Geometry check sheet. Reference: the model listing, model coordinates, mm. A direction names the side the tool comes from. Round coordinates to 2 decimals unless told otherwise and drop trailing zeros. Write each loop counter-clockwise with the first axis right and the second up, starting at its lowest first coordinate (ties: lowest second). Pieces come first, ordered by that corner, then holes. Notation, with made-up numbers: M -6,83 L 45,83 A5 ccw 45,88 Z; hole C 80,50.25 d5. An arc over 180 degrees is marked long. Use a Markdown table: item, result.
Autodesk Inventor part; units mm, degrees
ref_plane "Work Plane1" through (1.525, 0, 0) normal (0, 0, 1) x (1, 0, 0)
ref_plane "YZ Plane" through (0, 0, 0) normal (1, 0, 0) x (0, 1, 0)
ref_plane "XZ Plane" through (0, 0, 0) normal (0, 1, 0) x (-1, 0, 0)
sketch "Sketch1" plane through (0, 0, 0) normal (0, 0, 1) x (1, 0, 0)
  line L0 (0, 7.1374) -> (0, 4.9276)
  line L1 (101.6, 4.7625) -> (127, 4.7625)
  line L2 (127, 4.7625) -> (127, 0)
  line L3 (127, 0) -> (-0.0001, 0)
  line L4 (-25.4001, 0) -> (152.4, 0)
  line L5 (-0.0001, 0) -> (-0.0001, 7.1374)
  line L6 (-0.0001, 7.1374) -> (0, 7.1374)
  line L7 (101.6, 4.7625) -> (97.6311, 4.9276)
  line L8 (97.6311, 4.9276) -> (0, 4.9276)
  line L9 (0, -1.4275) -> (0, 8.5649)
  dimension "d0" = 127
  dimension "d1" = 25.4
  dimension "d2" = 9.525
  dimension "d9" = 0.0001
  dimension "d10" = 14.2748
  dimension "d13" = 3.9689
  dimension "d14" = 9.8552
revolve "Body" add sketch "Sketch1" angle 360 about axis through (127, 0, 0) along (-1, 0, 0)
sketch "Sketch2" plane through (-0.0001, 0, 0) normal (-1, 0, 0) x (0, 0, 1)
  line L0 (0, 8.2416) -> (7.1374, 4.1208)
  line L1 (7.1374, 4.1208) -> (7.1374, -4.1208)
  line L2 (7.1374, -4.1208) -> (0, -8.2416)
  line L3 (0, -8.2416) -> (-7.1374, -4.1208)
  line L4 (-7.1374, -4.1208) -> (-7.1374, 4.1208)
  line L5 (-7.1374, 4.1208) -> (0, 8.2416)
  point P0 (0, 0)
  point P1 (0, 0)
  dimension "d11" = 14.2748
extrude "Head" add sketch "Sketch2" along normal blind 6.8072
sketch "Sketch4" plane through (0, 0, 0) normal (0, 0, 1) x (1, 0, 0)
  line L0 (-6.8073, 7.1374) -> (-6.8073, 8.2416)
  line L1 (-6.8073, 8.2416) -> (-6.1698, 8.2416)
  line L2 (-6.1698, 8.2416) -> (-6.8073, 7.1374)
  line L3 (-8.1687, 0) -> (1.3613, 0)
  line L4 (-0.0001, 8.2416) -> (-6.8073, 8.2416)
  line L5 (-6.8073, 4.1208) -> (-6.8073, 8.2416)
  dimension "d5" = 30
  dimension "d19" = 14.2748
revolve "Chamfer1" cut sketch "Sketch4" angle 360 about axis through (-10, 0, 0) along (1, 0, 0)
thread "Thread"
chamfer "Chamfer2" distance 0.9739 distance2 0.9447 1 edges at (127, -4.7625, 0) measured on face at (127, -1.1883, 1.0527)
ref_plane "Work Plane1" through (1.525, 0, 0) normal (0, 0, 1) x (1, 0, 0)
fillet "Fillet2" radius 0.762 1 edges at (0, -4.9276, 0)
equation "\"d0\" = NLG"
equation "\"d1\" = GEL"
equation "\"d2\" = GD"
equation "\"d10\" = SD2"
equation "\"d14\" = BDM"
equation "\"d11\" = SW"
equation "\"d3\" = KOH - SD"
equation "\"d5\" = ANG1"
equation "\"d19\" = SW0"
equation "\"d63\" = R"
equation "\"d15\" = GEL"
equation "\"d6\" = -0.5 * SPD + 0.5 * GD"
equation "\"NLG\" = 127"
equation "\"GD\" = NND"
equation "\"BDM\" = 9.8552"
equation "\"KOH\" = 6.8072"
equation "\"GEL\" = 25.4"
equation "\"SW\" = 14.2748"
equation "\"SW0\" = SW"
equation "\"SPD\" = GD1"
equation "\"SD2\" = SW"
equation "\"SD\" = 0"
equation "\"ANG1\" = 30deg"
equation "\"GAL\" = 3.96875"
equation "\"GUL\" = 0.238 * GAL"
equation "\"R\" = 0.762"
equation "\"d62\" = -NLG - SD + GUL"
equation "\"GD1\" = 7.5773"
equation "\"THREADDIA\" = 9.525"
equation "\"TOA\" = 30deg"
equation "\"NND\" = 9.525"
equation "\"E0\" = 1.155 * SW"
properties part number "ANSI/ASME B18.2.1 - 3/8-16 UNC - 5, HBI" material "Steel, Mild"
Item 1: Cross-section at B-B, the plane x = 111. Record the cut outline in (y, z) (1 decimal).
Outcome:
| item | result |
|---|---|
| outline | C 0,0 d9.5 |
Item 2: Access from +Z, -Z, +X, -X, +Y, -Y to the whole of each face (thin tool, end or side, straight path). Record for faces 1 (the face through (48.518, -4.923, -0.217)), 2 (the face through (-3.36, 6.15, -3.62)).
Outcome:
| item | result |
|---|---|
| face 1 | +X |
| face 2 | -Z, +X, -X, +Y |
Item 3: Cross-section at A-A, the plane x = 53.5. Record the cut outline in (y, z).
Outcome:
| item | result |
|---|---|
| outline | C 0,0 d9.86 |
Item 4: Go/stop test with flat-tipped pins: pin 1 (4 mm diameter, centred on y = -5.5, z = -2, fed in from +X); pin 2 (1.5 mm diameter, centred on y = -4, z = -3.5, fed in from +X); pin 3 (2 mm diameter, centred on x = 48, y = 2.5, fed in from +Z). Record where each tip stops, or that it passes through.
Outcome:
| item | result |
|---|---|
| pin 1 | stops at x = 126.94 |
| pin 2 | stops at x = 126.25 |
| pin 3 | stops at z = 4.69 |
Item 5: Material ranges on line 1 along Z through (x, y) = (9.5, 1.25); line 2 along Z through (x, y) = (113, 0.5); line 3 along X through (y, z) = (-4, -4.5), recorded low to high. Write a range as from..to.
Outcome:
| item | result |
|---|---|
| line 1 | z = -4.77..4.77 |
| line 2 | z = -4.74..4.74 |
| line 3 | x = -6.81..0 |
